Geometry check sheet. Reference: drawing and pictorial views, mm from the part's lowest x, y, z. A direction names the side the tool comes from. Give positions to 0.01 mm unless a question says otherwise; leave off trailing zeros. Write each loop counter-clockwise with the first axis right and the second up, starting at its lowest first coordinate (ties: lowest second). Pieces come first, ordered by that corner, then holes. Notation, with made-up numbers: (-34, 11) -> (13, 11) arc R34 ccw to (13, 50) -> close; hole circle Ø4 at (-20, -11.5). An arc over 180 degrees is marked (long way). Answer as CSV lines item,"result".
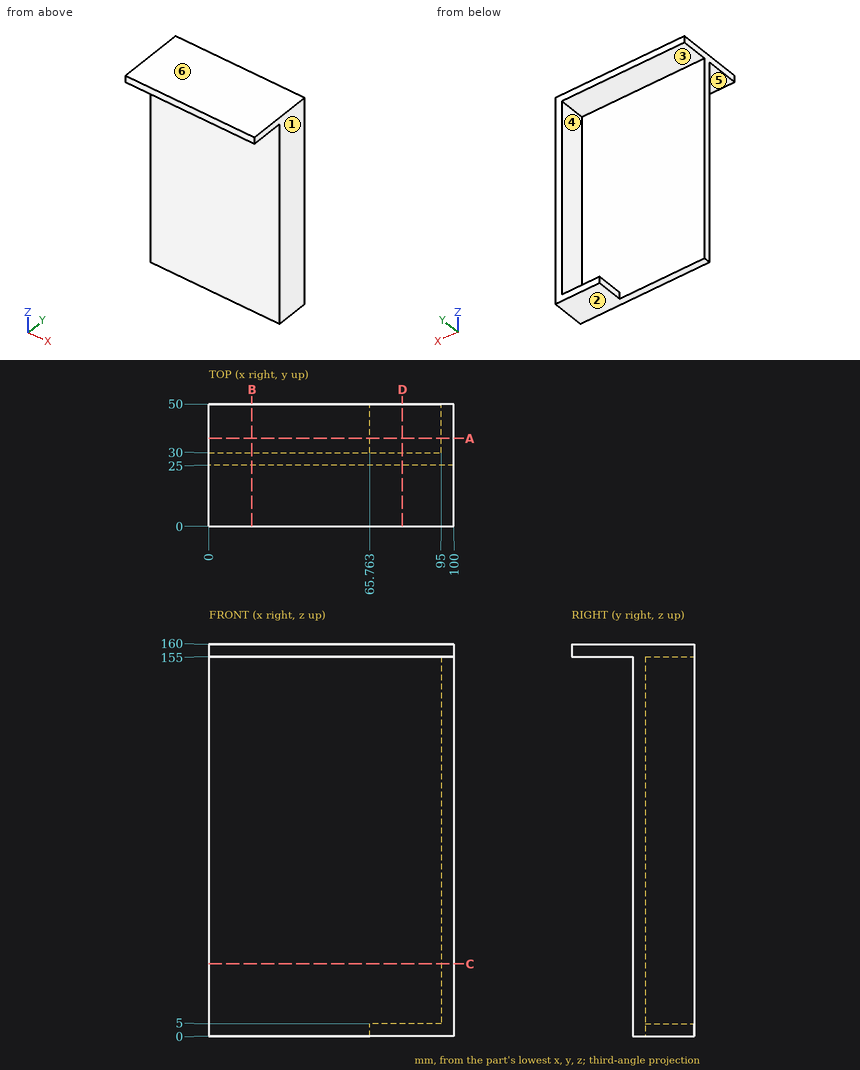
1) Scan lines: line 1 along Z through (x, y) = (94, 32); line 2 along Z through (x, y) = (14.5, 33.5); line 3 along Y through (x, z) = (21.5, 122.5). Record each from-to range of solid material in increasing order.
Reported:
line 1,"0 to 5, 155 to 160"
line 2,"155 to 160"
line 3,"25 to 30"
2) Depth check by flat-ended pin: pin 1 (6 mm diameter, centred on x = 63, z = 63.5, fed in from -Y); pin 2 (1.5 mm diameter, centred on y = 42, z = 2.5, fed in from -X); pin 3 (6 mm diameter, centred on y = 37.5, z = 49.5, fed in from -X). Enter the tip coordinate at first touch or a pass-through.
Reported:
pin 1,"y = 25"
pin 2,"x = 65.76"
pin 3,"x = 95"
3) Section check D-D (x = 79). Record the boundary of the cut face in (y, z), and give its area (4 significant figures).
Reported:
outline,"(0, 155) -> (25, 155) -> (25, 0) -> (50, 0) -> (50, 5) -> (30, 5) -> (30, 155) -> (50, 155) -> (50, 160) -> (0, 160) -> close"
area,"1,125 mm²"
4) Section check C-C (z = 29.5). Record the boundary of the cut face in (x, y).
Reported:
outline,"(0, 25) -> (100, 25) -> (100, 50) -> (95, 50) -> (95, 30) -> (0, 30) -> close"
5) Tool access check on the marked faces 4, 5 and 6. Record the directions out of +Z, -Z, +X, -X, +Y, -Y that give a thin tool (end or side, any length) a straight path to the whole face; none if there is none.
Reported:
face 4,"-X, +Y"
face 5,"-Z, +X, -X, -Y"
face 6,"+Z, +X, -X, +Y, -Y"
6) Section check B-B (x = 17.5). Record the boundary of the cut face in (y, z).
Reported:
outline,"(0, 155) -> (25, 155) -> (25, 0) -> (30, 0) -> (30, 155) -> (50, 155) -> (50, 160) -> (0, 160) -> close"
7) Draft check along Z on the marked faces 1, 2 and 3. Enter one of: +Z half, -Z half, draft (parallel to the pull), parting line (faces both ways), or undercut.
Reported:
face 1,"draft"
face 2,"-Z half"
face 3,"undercut"
8) Section check A-A (y = 36). Record the boundary of the cut face in (x, z).
Reported:
outline,"(0, 155) -> (95, 155) -> (95, 5) -> (65.76, 5) -> (65.76, 0) -> (100, 0) -> (100, 160) -> (0, 160) -> close"
